Part model, mm, in its own coordinate system. Face numbers are marked on the shaded views. A direction names the side the tool comes from. Give positions to 0.01 mm unless a question says otherwise; leave off trailing zeros. Order: outer loops, then holes, each group sorted by start corner. A loop starts at its lowest first (then second) coordinate and runs counter-clockwise, first axis right, second up. Notation, with made-up numbers: (80, -26.5) -> (118, -26.5) arc R17 cw to (118, 4.5) -> close; hole circle Ø8 at (42.5, 30). An arc over 180 degrees is marked (long way). Write item = value, one per line. Start each with the question number.
(1) Two-plate mould, pull along X, no slides. Class the marked faces 4, 5 and 6: pulls with the +X half, pulls with the -X half, needs draft (parallel to the pull), parting line crosses it, or undercut.
(2) Flat gauge pins, fed straight in: pin 1 (4 mm diameter, centred on x = 30.5, z = 7.5, fed in from +Y); pin 2 (3 mm diameter, centred on y = 19.5, z = -16.5, fed in from -X); pin 3 (8 mm diameter, centred on y = 4, z = -40.5, fed in from -X). Where does each tip first touch, or does it go through?
(3) Saw through at C-C, the plane y = 21. List the corners of the cut face in (x, z).
(4) Which spindle directions (+Z, -Z, +X, -X, +Y, -Y) get a long thin tool onto all of the face, cutting with end or side? Do the marked faces 1, 2 and 3. Say none if no direction does.
(5) Probe line 1 along X through (y, z) = (27, 0); line 2 along X through (y, z) = (11, 0); line 3 along Z through (x, y) = (-9.5, 34.5). List the from-to ranges inside material, lowest first. Write a range as from..to.
(6) Saw through at A-A, the plane z = 0. List the corners of the cut face in (x, y).
(7) Saw through at B-B, the plane x = 0. List the corners of the cut face in (y, z).
(8) Saw through at D-D, the plane z = 39.5. List the corners of the cut face in (x, y).
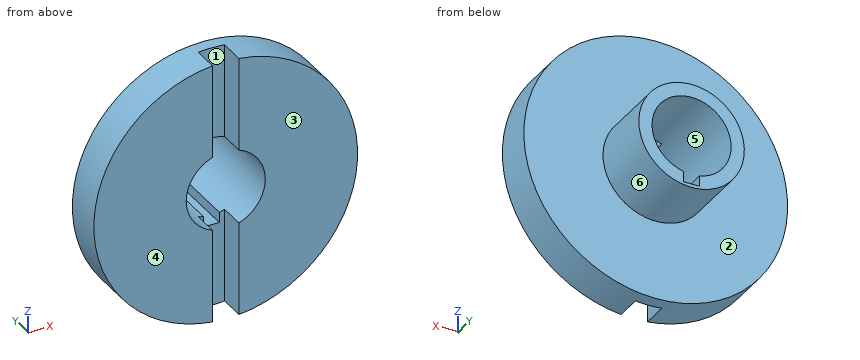
from build123d import *

# Parameters (mm, degrees)
SKETCH1_R           = 50
SKETCH1_R_2         = 20
BOSS_EXTRUDE1_DEPTH = 15
SKETCH1_3_R         = 20
BOSS_EXTRUDE2_DEPTH = 40
CUT_EXTRUDE1_DEPTH  = 10


with BuildPart() as part:
    # Sketch1 → Boss-Extrude1 (new body)
    with BuildSketch(Plane(origin=(0, 0, 0), x_dir=(1, 0, 0), z_dir=(0, 1, 0))):
        with Locations(Location((0, 0, 0), (0, 0, 270))):
            Circle(SKETCH1_R)
        with Locations(Location((0, 0, 0), (0, 0, 270))):
            Circle(SKETCH1_R_2, mode=Mode.SUBTRACT)
    extrude(amount=BOSS_EXTRUDE1_DEPTH)

    # Sketch1_3 → Boss-Extrude2 (add)
    with BuildSketch(Plane(origin=(0, 0, 0), x_dir=(1, 0, 0), z_dir=(0, 1, 0))):
        with Locations(Location((0, 0, 0), (0, 0, 270))):
            Circle(SKETCH1_3_R)
        with BuildLine():
            ThreePointArc((-3, 14.696938457), (0, -15), (3, 14.696938457))
            Line((3, 14.696938457), (3, 18.696938457))
            Line((3, 18.696938457), (-3, 18.696938457))
            Line((-3, 18.696938457), (-3, 14.696938457))
        make_face(mode=Mode.SUBTRACT)
    extrude(amount=BOSS_EXTRUDE2_DEPTH)

    # Sketch2 → Cut-Extrude1 (cut)
    with BuildSketch(Plane.XZ):
        with BuildLine():
            Line((-5, 49.749371855), (-5, -49.749371855))
            ThreePointArc((-5, -49.749371855), (0, -50), (5, -49.749371855))
            Line((5, -49.749371855), (5, 49.749371855))
            ThreePointArc((5, 49.749371855), (0, 50), (-5, 49.749371855))
        make_face()
    extrude(amount=-CUT_EXTRUDE1_DEPTH, mode=Mode.SUBTRACT)


solid = part.part
Results list:
q1.face_4 = needs draft
q1.face_5 = undercut
q1.face_6 = parting line crosses it
q2.pin_1 = 15
q2.pin_2 = -13.23
q2.pin_3 = -34.17
q3.outline = circle Ø40 at (0, 0); hole (-3, -18.7) -> (3, -18.7) -> (3, -14.7) arc R15 ccw (long way) to (-3, -14.7) -> close
q4.face_1 = +Z, -Z, -Y
q4.face_2 = +Y
q4.face_3 = +Z, -Z, +X, -X, -Y
q5.line_1 = -20..-15, 15..20
q5.line_2 = -50..-15, 15..50
q5.line_3 = -17.6..-11.61, 11.61..17.6
q6.outline = (-50, 0) -> (-15, 0) -> (-15, 40) -> (-20, 40) -> (-20, 15) -> (-50, 15) -> close; (15, 0) -> (50, 0) -> (50, 15) -> (20, 15) -> (20, 40) -> (15, 40) -> close
q7.outline = (10, -50) -> (15, -50) -> (15, -20) -> (40, -20) -> (40, -18.7) -> (10, -18.7) -> close; (10, 15) -> (40, 15) -> (40, 20) -> (15, 20) -> (15, 50) -> (10, 50) -> close
q8.outline = (-30.66, 0) -> (-5, 0) -> (-5, 10) -> (5, 10) -> (5, 0) -> (30.66, 0) -> (30.66, 15) -> (-30.66, 15) -> close
